Here's the drawing with two shaded views (mm, measured from the low corner). I have some questions. A direction names the side the tool comes from. Give positions to 0.01 mm unless a question says otherwise; leave off trailing zeros. Write each loop counter-clockwise with the first axis right and the second up, starting at its lowest first coordinate (ties: lowest second). Pieces come first, ordered by that corner, then holes. Notation, with made-up numbers: (-24, -15.75) - (24, -15.75) arc R28 ccw to (24, 2.25) - close; hole circle Ø9 at (-10, 15). An arc over 180 degrees is marked (long way). Use one line per item in the form item = value. Start each with the question number.
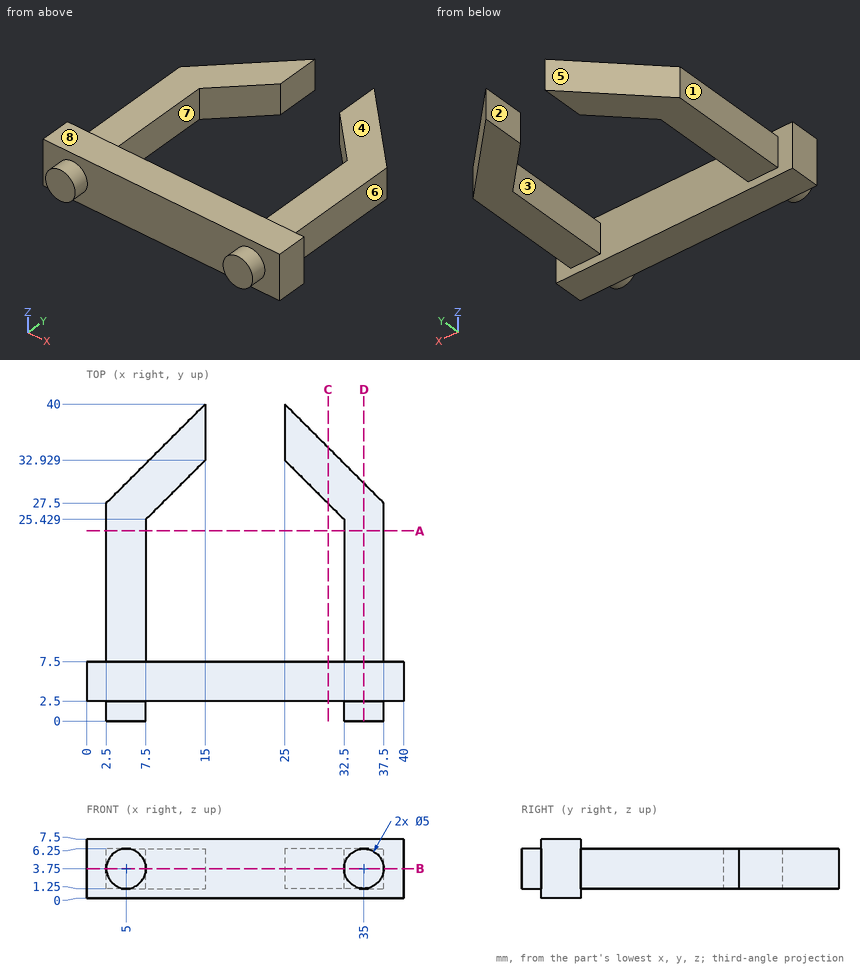
1. I want a section at A-A, the plane y = 24. List the corners of the cut face in (x, z) for me.
2. For the marked faces 1, 2, 3 and 4, which set-ups out of +Z, -Z, +X, -X, +Y, -Y let a thin tool reach every point of the face, with its end or its side?
3. I want a section at D-D, the plane x = 35. List the corners of the cut face in (y, z) for me.
4. I want a section at C-C, the plane x = 30.5. List the corners of the cut face in (y, z) for me.
5. For P1, Ø4, axis at y = 14.5, z = 4.5, coming from the +X side; P2, Ø4, axis at y = 36, z = 2.5, coming from the +X side; P3, Ø3, axis at y = 31, z = 5, coming from the -X side; P4, Ø1, axis at x = 23.5, y = 35.5, coming from the -Z side, each with a flat end and sliding along its axis, tell me the tip position at first contact or that it passes through.
6. Please list where these lines run through material, in increasing order: line 1 (Y direction, x = 17, z = 4.25); line 2 (X direction, y = 14.5, z = 4.5); line 3 (X direction, y = 26, z = 3).
7. I want a section at B-B, the plane z = 3.75. List the corners of the cut face in (x, y) for me, then the cut area to 3 significant figures.
8. We'd pull the mould along X, two halves only. Please class the marked faces 5, 6, 7 and 8: pulls with the +X half, pulls with the -X half, needs draft (parallel to the pull), parting line crosses it, or undercut.
Result sheet:
q1.outline = (2.5, 1.25) - (7.5, 1.25) - (7.5, 6.25) - (2.5, 6.25) - close; (32.5, 1.25) - (37.5, 1.25) - (37.5, 6.25) - (32.5, 6.25) - close
q2.face_1 = +Z, -Z, -X, +Y
q2.face_2 = +Z, -Z, +Y
q2.face_3 = +Z, -Z
q2.face_4 = +Z, +X, -X, +Y
q3.outline = (0, 1.25) - (2.5, 1.25) - (2.5, 0) - (7.5, 0) - (7.5, 1.25) - (30, 1.25) - (30, 6.25) - (7.5, 6.25) - (7.5, 7.5) - (2.5, 7.5) - (2.5, 6.25) - (0, 6.25) - close
q4.outline = (2.5, 0) - (7.5, 0) - (7.5, 7.5) - (2.5, 7.5) - close; (27.43, 1.25) - (34.5, 1.25) - (34.5, 6.25) - (27.43, 6.25) - close
q5.P1 = 37.5
q5.P2 = 31
q5.P3 = 4.5
q5.P4 = through
q6.line_1 = 2.5 to 7.5
q6.line_2 = 2.5 to 7.5, 32.5 to 37.5
q6.line_3 = 2.5 to 8.07, 31.93 to 37.5
q7.outline = (0, 2.5) - (2.5, 2.5) - (2.5, 0) - (7.5, 0) - (7.5, 2.5) - (32.5, 2.5) - (32.5, 0) - (37.5, 0) - (37.5, 2.5) - (40, 2.5) - (40, 7.5) - (37.5, 7.5) - (37.5, 27.5) - (25, 40) - (25, 32.93) - (32.5, 25.43) - (32.5, 7.5) - (7.5, 7.5) - (7.5, 25.43) - (15, 32.93) - (15, 40) - (2.5, 27.5) - (2.5, 7.5) - (0, 7.5) - close
q7.area = 556 mm2
q8.face_5 = pulls with the -X half
q8.face_6 = pulls with the +X half
q8.face_7 = undercut
q8.face_8 = needs draft
